Verification items for the finished model (mm, model axes). A direction names the side the tool comes from. Coordinates: 2 decimals unless noted, no trailing zeros. Loops run counter-clockwise (first coordinate to the right, second up) from the corner with the lowest first, then second, coordinate; pieces in that order, holes last. Notation, with made-up numbers: (-34.75, -33.75) -> (0.25, -33.75) arc R19 cw to (0.25, -0.75) -> close; hole circle Ø6 at (26.5, 5). An arc over 180 degrees is marked (long way). Use CSV: the item, a comma, the result in double quotes. Start each with the question number.
```python
from build123d import *

# Parameters (mm, degrees)
ESBO_O1_R                = 3
ESBO_O1_R_2              = 2
RESSALTO_EXTRUS_O1_DEPTH = 8.1
RESSALTO_EXTRUS_O2_DEPTH = 8.1
RESSALTO_EXTRUS_O3_DEPTH = 8.1
RESSALTO_EXTRUS_O4_START = -8.1
ESBO_O6_R                = 2
RESSALTO_EXTRUS_O4_DEPTH = 8.1
ESBO_O7_R                = 3
ESBO_O7_R_2              = 2
RESSALTO_EXTRUS_O5_DEPTH = 1.7


with BuildPart() as part:
    # Esboço1 → Ressalto-extrusão1 (new body)
    with BuildSketch(Plane.XY):
        Circle(ESBO_O1_R)
        Circle(ESBO_O1_R_2, mode=Mode.SUBTRACT)
    extrude(amount=RESSALTO_EXTRUS_O1_DEPTH)

    # Esboço2 → Ressalto-extrusão2 (add)
    with BuildSketch(Plane.XY):
        with BuildLine():
            Line((-2.958039892, 0.5), (-2.998801098, 0.5))
            Line((-2.998801098, 0.5), (-4.498801098, 0.5))
            Line((-4.498801098, 0.5), (-4.498801098, -0.5))
            Line((-4.498801098, -0.5), (-3, -0.5))
            Line((-3, -0.5), (-2.958039892, -0.5))
            ThreePointArc((-2.958039892, -0.5), (-2.989491568, -0.250878781), (-3, 0))
            ThreePointArc((-3, 0), (-2.989491568, 0.250878781), (-2.958039892, 0.5))
        make_face()
    extrude(amount=RESSALTO_EXTRUS_O2_DEPTH)

    # Esboço3 → Ressalto-extrusão3 (add)
    with BuildSketch(Plane(origin=(0, 0, 0), x_dir=(-1, 0, 0), z_dir=(0, 0, -1))):
        with BuildLine():
            ThreePointArc((0.5, -2.958039892), (0.250878781, -2.989491568), (0, -3))
            ThreePointArc((0, -3), (-0.250878781, -2.989491568), (-0.5, -2.958039892))
            Line((-0.5, -2.958039892), (-0.5, -4.458039892))
            Line((-0.5, -4.458039892), (0.5, -4.458039892))
            Line((0.5, -4.458039892), (0.5, -3))
            Line((0.5, -3), (0.5, -2.958039892))
        make_face()
        with BuildLine():
            ThreePointArc((-2.958039892, -0.5), (-2.989491568, -0.250878781), (-3, 0))
            ThreePointArc((-3, 0), (-2.989491568, 0.250878781), (-2.958039892, 0.5))
            Line((-2.958039892, 0.5), (-3, 0.5))
            Line((-3, 0.5), (-4.5, 0.5))
            Line((-4.5, 0.5), (-4.5, -0.5))
            Line((-4.5, -0.5), (-2.958039892, -0.5))
        make_face()
        with BuildLine():
            Line((0.5, 4.5), (0.5, 3))
            Line((0.5, 3), (0.5, 2.958039892))
            ThreePointArc((0.5, 2.958039892), (0, 3), (-0.5, 2.958039892))
            Line((-0.5, 2.958039892), (-0.5, 3))
            Line((-0.5, 3), (-0.5, 4.5))
            Line((-0.5, 4.5), (0.5, 4.5))
        make_face()
    extrude(amount=-RESSALTO_EXTRUS_O3_DEPTH)

    # Esboço6 → Ressalto-extrusão4 (add)
    # profile 1 of 5: a face of its own
    with BuildSketch(Plane.XY.offset(8.1).offset(RESSALTO_EXTRUS_O4_START)):
        with BuildLine():
            ThreePointArc((2.958039892, 0.5), (2.121320344, 2.121320344), (0.5, 2.958039892))
            ThreePointArc((0.5, 2.958039892), (0.00124461, 2.999999742), (-0.497545425, 2.958453743))
            ThreePointArc((-0.497545425, 2.958453743), (-0.498772755, 2.958247072), (-0.5, 2.958039892))
            ThreePointArc((-0.5, 2.958039892), (-2.121320344, 2.121320344), (-2.958039892, 0.5))
            ThreePointArc((-2.958039892, 0.5), (-3, 0), (-2.958039892, -0.5))
            ThreePointArc((-2.958039892, -0.5), (-2.121320344, -2.121320344), (-0.5, -2.958039892))
            ThreePointArc((-0.5, -2.958039892), (0, -3), (0.5, -2.958039892))
            ThreePointArc((0.5, -2.958039892), (2.121320344, -2.121320344), (2.958039892, -0.5))
            ThreePointArc((2.958039892, -0.5), (2.989491568, -0.250878781), (3, 0))
            ThreePointArc((3, 0), (2.989491568, 0.250878781), (2.958039892, 0.5))
        make_face()
        Circle(ESBO_O6_R, mode=Mode.SUBTRACT)
    # profile 2 of 5: a face of its own
    with BuildSketch(Plane.XY.offset(8.1).offset(RESSALTO_EXTRUS_O4_START)):
        with BuildLine():
            ThreePointArc((-0.497545425, 2.958453743), (0.00124461, 2.999999742), (0.5, 2.958039892))
            Line((0.5, 2.958039892), (0.5, 4.5))
            Line((0.5, 4.5), (-0.497545425, 4.5))
            Line((-0.497545425, 4.5), (-0.497545425, 2.958453743))
        make_face()
    # profile 3 of 5: a face of its own
    with BuildSketch(Plane.XY.offset(8.1).offset(RESSALTO_EXTRUS_O4_START)):
        with BuildLine():
            Line((4.5, 0.5), (2.958039892, 0.5))
            ThreePointArc((2.958039892, 0.5), (2.989491568, 0.250878781), (3, 0))
            ThreePointArc((3, 0), (2.989491568, -0.250878781), (2.958039892, -0.5))
            Line((2.958039892, -0.5), (4.5, -0.5))
            Line((4.5, -0.5), (4.5, 0.5))
        make_face()
    # profile 4 of 5: a face of its own
    with BuildSketch(Plane.XY.offset(8.1).offset(RESSALTO_EXTRUS_O4_START)):
        with BuildLine():
            Line((0.5, -4.458039892), (0.5, -2.958039892))
            ThreePointArc((0.5, -2.958039892), (0, -3), (-0.5, -2.958039892))
            Line((-0.5, -2.958039892), (-0.5, -4.458039892))
            Line((-0.5, -4.458039892), (0.5, -4.458039892))
        make_face()
    # profile 5 of 5: a face of its own
    with BuildSketch(Plane.XY.offset(8.1).offset(RESSALTO_EXTRUS_O4_START)):
        with BuildLine():
            ThreePointArc((-2.958039892, -0.5), (-3, 0), (-2.958039892, 0.5))
            Line((-2.958039892, 0.5), (-4.498801098, 0.5))
            Line((-4.498801098, 0.5), (-4.498801098, -0.5))
            Line((-4.498801098, -0.5), (-2.958039892, -0.5))
        make_face()
    extrude(amount=RESSALTO_EXTRUS_O4_DEPTH)

    # Esboço7 → Ressalto-extrusão5 (add)
    with BuildSketch(Plane.XY.offset(8.1)):
        with Locations(Location((0, 0, 0), (0, 0, 170.405931773))):
            Circle(ESBO_O7_R)
        Circle(ESBO_O7_R_2, mode=Mode.SUBTRACT)
    extrude(amount=RESSALTO_EXTRUS_O5_DEPTH)


solid = part.part
```
1. Depth check by flat-ended pin: pin 1 (1.7 mm diameter, centred on y = 3.5, z = 3, fed in from +X); pin 2 (0.8 mm diameter, centred on x = 4, z = 3, fed in from +Y); pin 3 (0.8 mm diameter, centred on x = 0, y = 3.5, fed in from +Z). Enter the tip coordinate at first touch or a pass-through.
2. Cross-section at C-C, the plane y = -1.5. Record the boundary of the cut face in (x, z), plus the area to 3 significant figures.
3. Cross-section at B-B, the plane z = 5.25. Record the boundary of the cut face in (x, y), plus the area to 3 significant figures.
4. Scan lines: line 1 (Y direction, x = 0, z = 2.75); line 2 (X direction, y = 1.75, z = 9.75); line 3 (X direction, y = -3.5, z = 3.5). Record each from-to range of solid material in increasing order.
5. Cross-section at D-D, the plane y = 0. Record the boundary of the cut face in (x, z).
6. Release check for a two-part mould opening along X. For faces 1 (the flat face through (-2, 1, 9.8)), 2 (the cylindrical face through (0, -2, 5)), 3 (the flat face through (-0.5, 4, 4)) record: released by +X, released by -X, zero draft, split by the parting line, or undercut.
7. Cross-section at A-A, the plane x = 0. Record the boundary of the cut face in (y, z).
8. Set-up check for faces 4 (the flat face through (4, -0.5, 4)), 5 (the flat face through (0.5, 4, 4)), 6 (the flat face through (-0.5, -4, 4)), 7 (the flat face through (-4, 0.5, 4)): record each of +Z, -Z, +X, -X, +Y, -Y from which the full face is reachable in a straight line by a thin tool's end or side.
Solution:
1,pin 1,"stops at x = 1.41"
1,pin 2,"stops at y = 0.5"
1,pin 3,"stops at z = 8.1"
2,outline,"(-2.6, 0) -> (-1.32, 0) -> (-1.32, 9.8) -> (-2.6, 9.8) -> close; (1.32, 0) -> (2.6, 0) -> (2.6, 9.8) -> (1.32, 9.8) -> close"
2,area,"25.0 mm2"
3,outline,"(-4.5, -0.5) -> (-2.96, -0.5) arc R3 ccw to (-0.5, -2.96) -> (-0.5, -4.46) -> (0.5, -4.46) -> (0.5, -2.96) arc R3 ccw to (2.96, -0.5) -> (4.5, -0.5) -> (4.5, 0.5) -> (2.96, 0.5) arc R3 ccw to (0.5, 2.96) -> (0.5, 4.5) -> (-0.5, 4.5) -> (-0.5, 2.96) arc R3 ccw to (-2.96, 0.5) -> (-4.5, 0.5) -> close; hole circle Ø4 at (0, 0)"
3,area,"21.7 mm2"
4,line 1,"y = -4.46 to -2, 2 to 4.5"
4,line 2,"x = -2.44 to -0.97, 0.97 to 2.44"
4,line 3,"x = -0.5 to 0.5"
5,outline,"(-4.5, 0) -> (-2, 0) -> (-2, 9.8) -> (-3, 9.8) -> (-3, 8.1) -> (-4.5, 8.1) -> close; (2, 0) -> (4.5, 0) -> (4.5, 8.1) -> (3, 8.1) -> (3, 9.8) -> (2, 9.8) -> close"
6,face 1,"zero draft"
6,face 2,"undercut"
6,face 3,"released by -X"
7,outline,"(-4.46, 0) -> (-2, 0) -> (-2, 9.8) -> (-3, 9.8) -> (-3, 8.1) -> (-4.46, 8.1) -> close; (2, 0) -> (4.5, 0) -> (4.5, 8.1) -> (3, 8.1) -> (3, 9.8) -> (2, 9.8) -> close"
8,face 4,"+Z, -Z, +X, -Y"
8,face 5,"+Z, -Z, +X, +Y"
8,face 6,"+Z, -Z, -X, -Y"
8,face 7,"+Z, -Z, -X, +Y"
